Can you work these out from the drawing? Everything is in mm from the part's minimum corner. A direction names the side the tool comes from. Coordinates: 2 decimals unless noted, no trailing zeros. Write each loop counter-clockwise with the first axis right and the second up, starting at its lowest first coordinate (ties: lowest second). Pieces come first, ordered by that corner, then holes. Notation, with made-up numbers: M -7.75,64 L 6.25,64 A12 cw 6.25,72 Z; hole C 51,40 d2. An arc over 180 degrees is marked long. Write item = value, one per line.
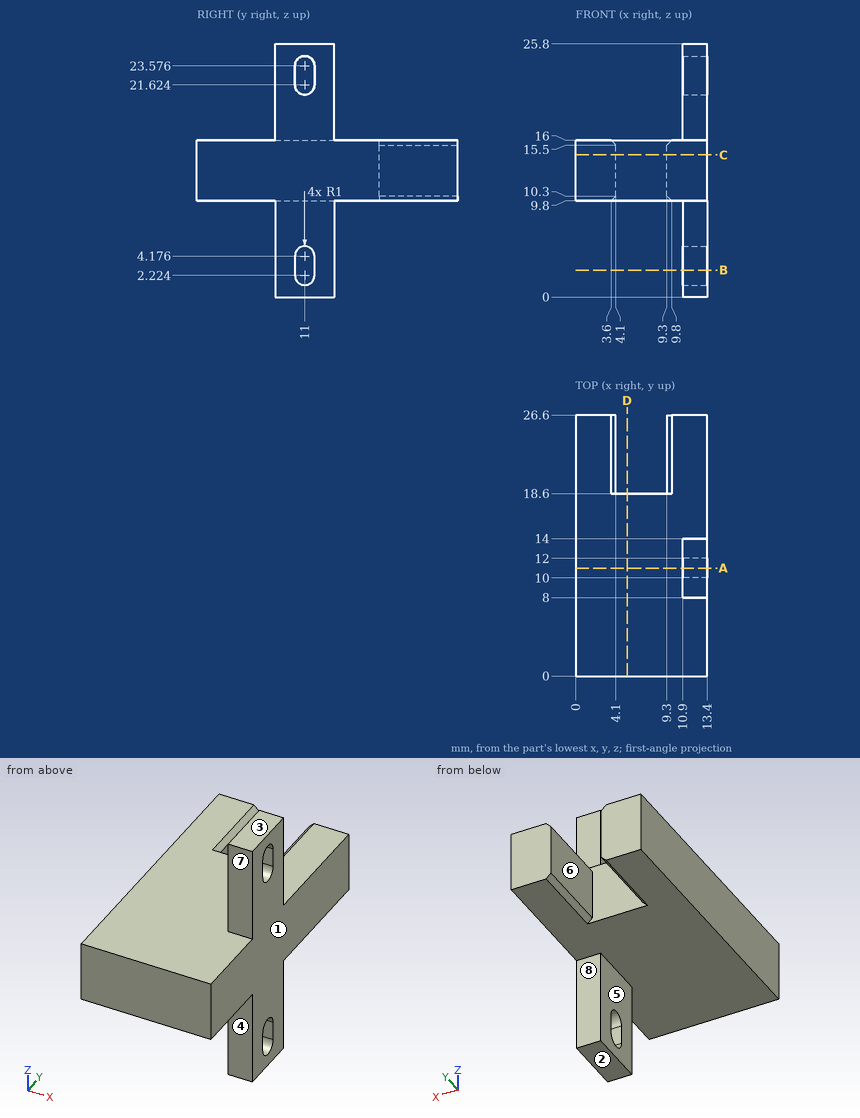
Item 1: I'm going to push flat-ended pins straight in: P1, Ø6.5, axis at y = 10, z = 4, coming from the -X side; P2, Ø2, axis at x = 12, z = 20, coming from the -Y side; P3, Ø12, axis at y = 6, z = 9, coming from the -X side; P4, Ø4, axis at x = 7.5, y = 18, coming from the +Z side. Where does each tip first touch, or does it pass through?
Numbers:
P1 = 10.9
P2 = 8
P3 = 0
P4 = 16
Item 2: Imagine slicing it at A-A (y = 11). Write out the boundary of the cut face in (x, z), and give its area (3 significant figures).
Numbers:
outline = M 0,9.8 L 10.9,9.8 L 10.9,5.18 L 13.4,5.18 L 13.4,20.62 L 10.9,20.62 L 10.9,16 L 0,16 Z; M 10.9,0 L 13.4,0 L 13.4,1.22 L 10.9,1.22 Z; M 10.9,24.58 L 13.4,24.58 L 13.4,25.8 L 10.9,25.8 Z
area = 112 mm²
Item 3: Imagine slicing it at D-D (x = 5.25). Write out the boundary of the cut face in (y, z), and give its area (3 significant figures).
Numbers:
outline = M 0,9.8 L 18.6,9.8 L 18.6,16 L 0,16 Z
area = 115 mm²
Item 4: For the marked faces 4, 5, 6, 7 and 8, which set-ups out of +Z, -Z, +X, -X, +Y, -Y let a thin tool reach every point of the face, with its end or its side?
Numbers:
face_4 = -Z, +X, -X, -Y
face_5 = -Z, -X, +Y, -Y
face_6 = +Z, -Z, +Y
face_7 = +Z, +X, -X, -Y
face_8 = -Z, +X, -X, +Y
Item 5: Imagine slicing it at B-B (z = 2.75). Write out the boundary of the cut face in (x, y).
Numbers:
outline = M 10.9,8 L 13.4,8 L 13.4,10 L 10.9,10 Z; M 10.9,12 L 13.4,12 L 13.4,14 L 10.9,14 Z
Item 6: Imagine slicing it at C-C (z = 14.5). Write out the boundary of the cut face in (x, y).
Numbers:
outline = M 0,0 L 13.4,0 L 13.4,26.6 L 9.3,26.6 L 9.3,18.6 L 4.1,18.6 L 4.1,26.6 L 0,26.6 Z
Item 7: If I drill on line 1 along Z through (x, y) = (12.75, 11); line 2 along Y through (x, z) = (11, 3.5); line 3 along Z through (x, y) = (10.75, 16.5), over which ranges is the centre line in solid material (lowest first)?
Numbers:
line_1 = 0 to 1.22, 5.18 to 20.62, 24.58 to 25.8
line_2 = 8 to 10, 12 to 14
line_3 = 9.8 to 16
Item 8: If we mould it in two halves opening along Z, with no side actions, what happens to the marked faces 1, 2 and 3? For each: pulls with the +Z half, pulls with the -Z half, needs draft (parallel to the pull), parting line crosses it, or undercut.
Numbers:
face_1 = needs draft
face_2 = pulls with the -Z half
face_3 = pulls with the +Z half
